```python
from build123d import *

# Parameters (mm, degrees)
SKETCH1_W                = 91.4
SKETCH1_H                = 68.6
BOSS_EXTRUDE1_DEPTH      = 1.7
BOSS_EXTRUDE2_START      = 4
SKETCH2_R                = 20
BOSS_EXTRUDE2_DEPTH      = 11
SKETCH3_R                = 4
BOSS_EXTRUDE3_DEPTH      = 10.5
SKETCH4_W                = 10
SKETCH4_H                = 10
BOSS_EXTRUDE4_DEPTH      = 3.8
SKETCH6_R                = 10
BOSS_EXTRUDE5_DEPTH      = 15
SKETCH7_W                = 6.8
SKETCH7_H                = 9.7
SKETCH7_W_2              = 9.7
SKETCH7_H_2              = 3.8
BOSS_EXTRUDE6_DEPTH      = 9.7
SKETCH8_W                = 24
SKETCH8_H                = 5.5
SKETCH8_W_2              = 5.5
SKETCH8_H_2              = 24
SKETCH8_H_3              = 16
SKETCH8_W_3              = 12
SKETCH8_W_4              = 10
SKETCH8_W_5              = 16
BOSS_EXTRUDE7_DEPTH      = 7
SKETCH9_W                = 7
SKETCH9_H                = 7
BOSS_EXTRUDE8_DEPTH      = 5.9
M3_CLEARANCE_HOLE1_D     = 3.6
M3_CLEARANCE_HOLE1_DEPTH = 7.5
M3_CLEARANCE_HOLE1_TIP   = 1.081549114
FILLET1_SIZE             = 3
CUT_EXTRUDE1_START       = -2.25
SKETCH12_R               = 20
SKETCH12_R_2             = 18
CUT_EXTRUDE1_DEPTH       = 1
LPATTERN1_COUNT          = 4
LPATTERN1_PITCH          = 2.5


with BuildPart() as part:
    # Sketch1 → Boss-Extrude1 (new body)
    with BuildSketch(Plane(origin=(0, 0, 0), x_dir=(1, 0, 0), z_dir=(0, 1, 0))):
        Rectangle(SKETCH1_W, SKETCH1_H)
    extrude(amount=BOSS_EXTRUDE1_DEPTH)

    # Sketch3 → Boss-Extrude3 (add)
    with BuildSketch(Plane(origin=(0, 1.7, 0), x_dir=(1, 0, 0), z_dir=(0, 1, 0))):
        with Locations(Location((24.5, 27.4, 0), (0, 0, 90))):
            Circle(SKETCH3_R)
        with Locations(Location((33.7, 27.4, 0), (0, 0, 90))):
            Circle(SKETCH3_R)
        with Locations(Location((33.7, -27.4, 0), (0, 0, 90))):
            Circle(SKETCH3_R)
        with Locations(Location((24.5, -27.4, 0), (0, 0, 90))):
            Circle(SKETCH3_R)
    extrude(amount=BOSS_EXTRUDE3_DEPTH)

    # Sketch4 → Boss-Extrude4 (add)
    with BuildSketch(Plane(origin=(0, 1.7, 0), x_dir=(1, 0, 0), z_dir=(0, 1, 0))):
        with Locations((27.7, 5.5)):
            Rectangle(SKETCH4_W, SKETCH4_H)
        with Locations((27.7, 16.5)):
            Rectangle(SKETCH4_W, SKETCH4_H)
        with Locations((27.7, -5.5)):
            Rectangle(SKETCH4_W, SKETCH4_H)
        with Locations((27.7, -16.5)):
            Rectangle(SKETCH4_W, SKETCH4_H)
    extrude(amount=BOSS_EXTRUDE4_DEPTH)



with BuildPart() as body_2:
    # Sketch2 → Boss-Extrude2 (new body)
    with BuildSketch(Plane(origin=(0, 1.7, 0), x_dir=(1, 0, 0), z_dir=(0, 1, 0)).offset(BOSS_EXTRUDE2_START)):
        with Locations(Location((3.7, 0, 0), (0, 0, 270))):
            Circle(SKETCH2_R)
    extrude(amount=BOSS_EXTRUDE2_DEPTH)


with BuildPart() as part_1:
    add(part.part)

    add(body_2.part)  # Boss-Extrude5 merges body 2
    # Sketch6 → Boss-Extrude5 (add)
    with BuildSketch(Plane(origin=(0, 16.7, 0), x_dir=(1, 0, 0), z_dir=(0, 1, 0))):
        with Locations(Location((3.7, 0, 0), (0, 0, 270))):
            Circle(SKETCH6_R)
    extrude(amount=-BOSS_EXTRUDE5_DEPTH)

    # Sketch7 → Boss-Extrude6 (add)
    with BuildSketch(Plane(origin=(0, 1.7, 0), x_dir=(1, 0, 0), z_dir=(0, 1, 0))):
        with Locations((39.2, 0)):
            Rectangle(SKETCH7_W, SKETCH7_H)
        with Locations((-29.25, 31.55)):
            Rectangle(SKETCH7_W_2, SKETCH7_H_2)
    extrude(amount=BOSS_EXTRUDE6_DEPTH)

    # Sketch8 → Boss-Extrude7 (add)
    with BuildSketch(Plane(origin=(0, 1.7, 0), x_dir=(1, 0, 0), z_dir=(0, 1, 0))):
        with Locations((7.6, -31.35)):
            Rectangle(SKETCH8_W, SKETCH8_H)
        with Locations((-42.75, 14.7)):
            Rectangle(SKETCH8_W_2, SKETCH8_H_2)
        with Locations((-42.75, -6.3)):
            Rectangle(SKETCH8_W_2, SKETCH8_H_3)
        with Locations((-15.3, 31.35)):
            Rectangle(SKETCH8_W_3, SKETCH8_H)
        with Locations((-3.3, 31.35)):
            Rectangle(SKETCH8_W_4, SKETCH8_H)
        with Locations((10.7, 31.35)):
            Rectangle(SKETCH8_W_5, SKETCH8_H)
    extrude(amount=BOSS_EXTRUDE7_DEPTH)

    # Sketch9 → Boss-Extrude8 (add)
    with BuildSketch(Plane(origin=(0, 1.7, 0), x_dir=(1, 0, 0), z_dir=(0, 1, 0))):
        with Locations((-33.7, -30.3)):
            Rectangle(SKETCH9_W, SKETCH9_H)
        with Locations((-25.366666667, -30.3)):
            Rectangle(SKETCH9_W, SKETCH9_H)
        with Locations((-17.033333333, -30.3)):
            Rectangle(SKETCH9_W, SKETCH9_H)
        with Locations((-8.7, -30.3)):
            Rectangle(SKETCH9_W, SKETCH9_H)
    extrude(amount=BOSS_EXTRUDE8_DEPTH)

    # M3 Clearance Hole1
    with Locations(Plane(origin=(0, 1.7, 0), x_dir=(1, 0, 0), z_dir=(0, 1, 0))):
        with Locations((41.7, 30.3), (-41.7, -30.3), (41.7, -30.3), (-41.7, 30.3)):
            Hole(M3_CLEARANCE_HOLE1_D / 2, depth=M3_CLEARANCE_HOLE1_DEPTH)
            with Locations((0, 0, -(M3_CLEARANCE_HOLE1_DEPTH + M3_CLEARANCE_HOLE1_TIP / 2))):  # 118° drill point
                Cone(0, M3_CLEARANCE_HOLE1_D / 2, M3_CLEARANCE_HOLE1_TIP, mode=Mode.SUBTRACT)

    # Fillet1
    # a fillet whose section is not a circle: 3 mm, written as the material it takes off along each edge
    with BuildSketch(Plane(origin=(-45.7, -7.5, 34.3), x_dir=(1, 0, 0), z_dir=(0, 1, 0)), Plane(origin=(-45.7, -7.5, -34.3), x_dir=(0, 0, 1), z_dir=(0, 1, 0))) as fillet1_piece_1:
        with BuildLine():
            add(Edge.make_bspline([(FILLET1_SIZE, 0), (FILLET1_SIZE * 0.831801948466, 0), (FILLET1_SIZE * 0.663603896932, 0), (FILLET1_SIZE * 0.292893218813, FILLET1_SIZE * 0.0716919198361), (FILLET1_SIZE * 0.0716919198361, FILLET1_SIZE * 0.292893218813), (0, FILLET1_SIZE * 0.663603896932), (0, FILLET1_SIZE * 0.831801948466), (0, FILLET1_SIZE)], knots=[0, 0, 0, 0, 0, 0, 0.5, 0.5, 1, 1, 1, 1, 1, 1], degree=5))
            Line((0, FILLET1_SIZE), (0, 0))
            Line((0, 0), (FILLET1_SIZE, 0))
        make_face()
    extrude(amount=16.7, mode=Mode.SUBTRACT)
    with BuildSketch(Plane(origin=(45.7, -7.5, -34.3), x_dir=(0, 0, 1), z_dir=(0, 1, 0)), Plane(origin=(45.7, -7.5, 34.3), x_dir=(-1, 0, 0), z_dir=(0, 1, 0))) as fillet1_piece_2:
        with BuildLine():
            add(Edge.make_bspline([(FILLET1_SIZE, 0), (FILLET1_SIZE * 0.831801948466, 0), (FILLET1_SIZE * 0.663603896932, 0), (FILLET1_SIZE * 0.292893218813, -FILLET1_SIZE * 0.0716919198361), (FILLET1_SIZE * 0.0716919198361, -FILLET1_SIZE * 0.292893218813), (0, -FILLET1_SIZE * 0.663603896932), (0, -FILLET1_SIZE * 0.831801948466), (0, -FILLET1_SIZE)], knots=[0, 0, 0, 0, 0, 0, 0.5, 0.5, 1, 1, 1, 1, 1, 1], degree=5))
            Line((0, -FILLET1_SIZE), (0, 0))
            Line((0, 0), (FILLET1_SIZE, 0))
        make_face()
    extrude(amount=16.7, mode=Mode.SUBTRACT)

    # Sketch12 → Cut-Extrude1 (cut)
    with BuildSketch(Plane(origin=(0, 16.7, 0), x_dir=(1, 0, 0), z_dir=(0, 1, 0)).offset(CUT_EXTRUDE1_START)):
        with Locations(Location((3.7, 0, 0), (0, 0, 270))):
            Circle(SKETCH12_R)
        with Locations(Location((3.7, 0, 0), (0, 0, 270))):
            Circle(SKETCH12_R_2, mode=Mode.SUBTRACT)
    cut_extrude1 = extrude(amount=CUT_EXTRUDE1_DEPTH, mode=Mode.SUBTRACT)

    # LPattern1: Cut-Extrude1 ×4
    with Locations(*[(0, -i * LPATTERN1_PITCH, 0) for i in range(1, LPATTERN1_COUNT)]):
        add(cut_extrude1, mode=Mode.SUBTRACT)


solid = part_1.part
```
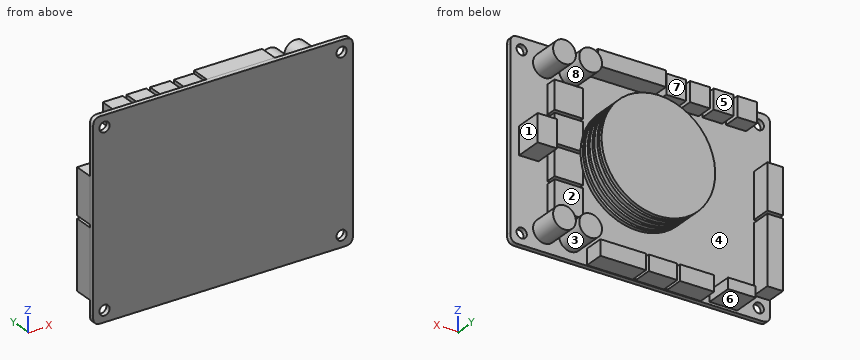
Check sheet for the modelled part. Datum: model origin and axes. Units: mm. Face numbers are marked on the shaded views. A direction names the side the tool comes from. Round coordinates to 2 decimals unless told otherwise and drop trailing zeros. Order: outer loops, then holes, each group sorted by start corner. A loop starts at its lowest first (then second) coordinate and runs counter-clockwise, first axis right, second up. Notation, with made-up numbers: (-14.75, 58) - (30.25, 58) arc R12 ccw to (30.25, 66) - close; hole circle Ø7 at (86.25, 75.5). An arc over 180 degrees is marked (long way). Write item = value, one per line.
Q1. Thickness scan on line 1 along X through (y, z) = (0.7, 30.3); line 2 along Z through (x, y) = (-41.7, 0.3); line 3 along Y through (x, z) = (9.5, 14). Record the ranges inside material, lowest first.
Computed:
line_1 = -45.7 to -43.5, -39.9 to 39.9, 43.5 to 45.7
line_2 = -34.3 to -32.1, -28.5 to 28.5, 32.1 to 34.3
line_3 = 0 to 1.7, 5.7 to 16.7
Q2. Tool access check on the marked faces 1, 2, 3, 4 and 5. Record the directions out of +Z, -Z, +X, -X, +Y, -Y that give a thin tool (end or side, any length) a straight path to the whole face; none if there is none.
Computed:
face_1 = +Z, -Z, +X, +Y
face_2 = +X, +Y
face_3 = +Y
face_4 = none
face_5 = +Z, -X, +Y
Q3. Section check A-A (x = -41.7). Record the boundary of the cut face in (y, z), and give its area (3 significant figures).
Computed:
outline = (0, -34.3) - (1.7, -34.3) - (1.7, -32.1) - (0, -32.1) - close; (0, -28.5) - (1.7, -28.5) - (1.7, -26.7) - (8.7, -26.7) - (8.7, -2.7) - (1.7, -2.7) - (1.7, -1.7) - (8.7, -1.7) - (8.7, 14.3) - (1.7, 14.3) - (1.7, 28.5) - (0, 28.5) - close; (0, 32.1) - (1.7, 32.1) - (1.7, 34.3) - (0, 34.3) - close
area = 384 mm^2
Q4. Draft check along Z on the marked faces 6, 7 and 8. Enter one of: pulls with the +Z half, pulls with the -Z half, needs draft (parallel to the pull), parting line crosses it, or undercut.
Computed:
face_6 = pulls with the -Z half
face_7 = needs draft
face_8 = undercut
Q5. Go/stop test with flat-tipped pins: pin 1 (4 mm diameter, centred on y = 6, z = 24, fed in from +X); pin 2 (10 mm diameter, centred on y = 13, z = -15, fed in from -X); pin 3 (3 mm diameter, centred on x = 13.5, z = 32, fed in from +Y); pin 4 (8 mm diameter, centred on x = -12.5, z = -25.5, fed in from -Y). Record where each tip stops, or that it passes through.
Computed:
pin_1 = 37.45
pin_2 = -45.5
pin_3 = 8.7
pin_4 = 0
Q6. Section check B-B (z = -25). Record the boundary of the cut face in (x, y), and give its area (3 significant figures).
Computed:
outline = (-45.7, 0) - (45.7, 0) - (45.7, 1.7) - (36.9, 1.7) - (36.9, 12.2) - (30.5, 12.2) - (30.5, 1.7) - (27.7, 1.7) - (27.7, 12.2) - (21.3, 12.2) - (21.3, 1.7) - (-40, 1.7) - (-40, 8.7) - (-45.5, 8.7) - (-45.5, 1.7) - (-45.7, 1.7) - close
area = 328 mm^2
